Build history of the part. All positions in model axes, mm. Coordinates: 2 decimals unless noted, no trailing zeros. Order: outer loops, then holes, each group sorted by start corner. A loop starts at its lowest first (then second) coordinate and runs counter-clockwise, first axis right, second up. Notation, with made-up numbers: M 62,-1 L 105,-1 A27 cw 105,31 Z; hole C 29.25,43.5 d3. An arc over 180 degrees is marked long. Write item = value, one per line. Start each with the question number.
Q1. Band-saw the part on D-D on x = -14. Write the cut outline in (y, z), plus the area to 3 significant figures.
Q2. Band-saw the part on A-A on x = 0. Write the cut outline in (y, z).
Q3. Band-saw the part on B-B on z = 0.7. Write the cut outline in (x, y).
Q4. Drill centre lines: probe 1 along X at (y, z) = (-20, 1.4); probe 2 along X at (y, z) = (-20.5, 1.7); probe 3 along Y at (x, z) = (-15, 0.9). Where is each one in solid material? Low to high.
Q5. Band-saw the part on C-C on y = -21. Write the cut outline in (x, z).
Q6. Pin check, flat tip, straight feed: P1, Ø5.5, axis at x = -14, y = -20, coming from the -Z side. Stop position of the tip, or through.
Autodesk Inventor part; units mm, degrees
ref_plane "YZ Plane" through (0, 0, 0) normal (1, 0, 0) x (0, 1, 0)
ref_plane "XZ Plane" through (0, 0, 0) normal (0, 1, 0) x (-1, 0, 0)
ref_plane "XY Plane" through (0, 0, 0) normal (0, 0, 1) x (1, 0, 0)
sketch "Sketch1" plane through (0, 0, 0) normal (0, 0, 1) x (1, 0, 0)
  circle A0 centre (16.2, 5) radius 9.025
  arc A1 (15.9625, 14.0219) -> (35.7029, 29.6112) centre (15.41, 35.0146) ccw
  arc A2 (8.6866, 0) -> (52.5133, -3.5421) centre (31.9968, 15.5125) ccw
  circle A3 centre (16.2, 5) radius 6.025
  arc A4 (70.0205, 42.4797) -> (35.7029, 29.6112) centre (57.4454, 23.8218) ccw
  circle A5 centre (14, -20) radius 3
  circle A6 centre (0, -20) radius 3
  circle A7 centre (-14, -20) radius 3
  line L0 (16.2, 5) -> (136.0469, 5) construction
  line L1 (16.2, 5) -> (120.1794, 65.0325) construction
  line L2 (16.2, 5) -> (136.265, 5) construction
  line L3 (16.2, 5) -> (121.2083, -55.6266) construction
  line L4 (16.2, 5) -> (137.4531, 5) construction
  arc A8 (11.4834, 12.6944) -> (20.7844, 36.0654) centre (0.5085, 30.5984) ccw construction
  arc A9 (7.1931, 4.4289) -> (43.377, -20.5519) centre (35.1365, 6.208) ccw construction
  arc A10 (11.4312, 12.7797) -> (21.4, 30) centre (0.5085, 30.5984) ccw
  line L5 (21.4, 30) -> (0, 30)
  arc A11 (7.0935, 4.4191) -> (25, -20) centre (35.1365, 6.208) ccw
  arc A12 (11.4312, 12.7797) -> (7.0935, 4.4191) centre (16.2, 5) ccw
  line L6 (0, 30) -> (0, -48.3313) construction
  line L7 (-21.4, 30) -> (0, 30)
  arc A13 (-21.4, 30) -> (-11.4312, 12.7797) centre (-0.5085, 30.5984) ccw
  arc A14 (-7.0935, 4.4191) -> (-11.4312, 12.7797) centre (-16.2, 5) ccw
  arc A15 (-25, -20) -> (-7.0935, 4.4191) centre (-35.1365, 6.208) ccw
  line L8 (-36.0984, -20) -> (40.4938, -20)
  circle A16 centre (23.9178, -22.798) radius 3
  circle A17 centre (-23.9178, -22.798) radius 3
  arc A18 (-24.9888, -25.6003) -> (24.9888, -25.6003) centre (0, 39.7874) ccw
  line L9 (-31.4755, -75) -> (165.3406, -75) construction
  point P0 (0, 0)
  point P1 (25.2806, -20)
  point P2 (-25.2806, -20)
  point P3 (-20.9441, -22.4019)
  point P4 (28.425, 18.534)
  dimension "d0" = 6
  dimension "d1" = 6
  dimension "d2" = 6
  dimension "d3" = 30
  dimension "d4" = 30
  dimension "d5" = 0.1
  dimension "d6" = 0.1
  dimension "d7" = 20.9
  dimension "d8" = 9.125
  dimension "d9" = 30
  dimension "d10" = 20
  dimension "d11" = 21.4
  dimension "d12" = 28
  dimension "d13" = 6
  dimension "d14" = 6
  dimension "d15" = 70
  dimension "d16" = 14
  dimension "d17" = 14
  dimension "d18" = 25
  dimension "d19" = 75
extrude "Extrusion1" add sketch "Sketch1" along normal blind 3 contours L8 A16 A18 A17 A7 A6 A5 | A5 L8 A6 A7 A17 A15 A14 A13 L7 L5 A10 A12 A11 A16 | A16 L8 | L8 A16 | A17 L8 | A17 L8
fillet "Fillet1" radius 2 2 edges at (21.4, 30, 1.5) (-21.4, 30, 1.5)
properties part number "中間ユニット外"
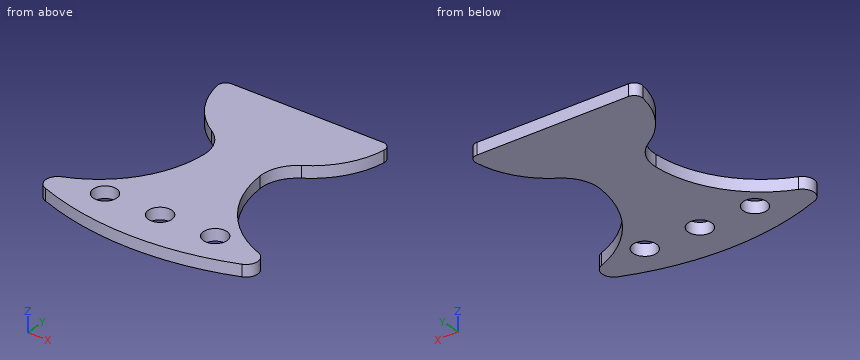
Recorded:
q1.outline = M -28.8,0 L -23,0 L -23,3 L -28.8,3 Z; M -17,0 L -12.31,0 L -12.31,3 L -17,3 Z; M 14.64,0 L 30,0 L 30,3 L 14.64,3 Z
q1.area = 77.6 mm2
q2.outline = M -30.21,0 L -23,0 L -23,3 L -30.21,3 Z; M -17,0 L 30,0 L 30,3 L -17,3 Z
q3.outline = M -25,-20 A3 ccw -24.99,-25.6 A70 ccw 24.99,-25.6 A3 ccw 25,-20 A28.1 cw 7.09,4.42 A9.13 cw 11.43,12.78 A20.9 ccw 21.21,27.73 A2 ccw 19.23,30 L -19.23,30 A2 ccw -21.21,27.73 A20.9 ccw -11.43,12.78 A9.12 cw -7.09,4.42 A28.1 cw Z; hole C -14,-20 d6; hole C 0,-20 d6; hole C 14,-20 d6
q4.probe_1 = -25 to -17, -11 to -3, 3 to 11, 17 to 25
q4.probe_2 = -25.85 to -16.96, -11.04 to -2.96, 2.96 to 11.04, 16.96 to 25.85
q4.probe_3 = -28.59 to -22.83, -17.17 to -13.39, 15.54 to 30
q5.outline = M -26.32,0 L -16.83,0 L -16.83,3 L -26.32,3 Z; M -11.17,0 L -2.83,0 L -2.83,3 L -11.17,3 Z; M 2.83,0 L 11.17,0 L 11.17,3 L 2.83,3 Z; M 16.83,0 L 26.32,0 L 26.32,3 L 16.83,3 Z
q6.P1 = through
